from build123d import *

# Parameters (mm, degrees)
SKETCH_1_W           = 2.4
SKETCH_1_H           = 2.4
EXTRUDE_1_DEPTH      = 7.2
EXTRUDE_2_DEPTH      = 18
EXTRUDE_2_DEPTH_BACK = 12
SKETCH_4_W           = 2.3
SKETCH_4_H           = 2.3
EXTRUDE_3_DEPTH      = 7
EXTRUDE_3_DEPTH_BACK = 2.3
SKETCH_5_R           = 0.35
SKETCH_6_R           = 0.35
CUT_EXTRUDE_1_DEPTH  = 10
FILLET_1_SIZE        = 2.4
FILLET_1_SIZE_2      = 3.2
FILLET_2_R           = 0.5
EXTRUDE_START        = -1.5
SKETCH_7_W           = 1.15
SKETCH_7_H           = 0.45
SKETCH_7_H_2         = 1.3
SKETCH_7_H_3         = 2.2
EXTRUDE_4_DEPTH      = 5.1
SKETCH_8_W           = 7.2
SKETCH_8_H           = 2.2
EXTRUDE_5_DEPTH      = 3.1


with BuildPart() as part:
    # 草图1 → 凸台-拉伸1 (new body)
    with BuildSketch(Plane.XY):
        Rectangle(SKETCH_1_W, SKETCH_1_H)
    extrude(amount=EXTRUDE_1_DEPTH)

    # 草图4 → 凸台-拉伸2 (add, two sides: drawn at the far end of the back side and taken through both)
    with BuildSketch(Plane(origin=(0, 0, 0), x_dir=(0, 0, -1), z_dir=(1, 0, 0)).offset(-EXTRUDE_2_DEPTH_BACK)):
        Rectangle(SKETCH_4_W, SKETCH_4_H)
    extrude(amount=EXTRUDE_2_DEPTH + EXTRUDE_2_DEPTH_BACK)

    # 草图5 → 凸台-拉伸3 (add, two sides: drawn at the far end of the back side and taken through both)
    with BuildSketch(Plane.XY.offset(1.15).offset(-EXTRUDE_3_DEPTH_BACK)):
        with BuildLine():
            Line((18, 0), (18, 1.15))
            Line((18, 1.15), (19.15, 1.15))
            ThreePointArc((19.15, 1.15), (20.3, 0), (19.15, -1.15))
            Line((19.15, -1.15), (18, -1.15))
            Line((18, -1.15), (18, 0))
        make_face()
        with Locations(Location((19.15, 0, 0), (0, 0, 180))):
            Circle(SKETCH_5_R, mode=Mode.SUBTRACT)
    extrude(amount=EXTRUDE_3_DEPTH + EXTRUDE_3_DEPTH_BACK)

    # 草图6 → 切除-拉伸1 (cut)
    with BuildSketch(Plane.ZY.offset(12)):
        Circle(SKETCH_6_R)
    extrude(amount=-CUT_EXTRUDE_1_DEPTH, mode=Mode.SUBTRACT)

    # 圆角1
    # an asymmetric fillet: 3.2, 2.4 mm, written as the material it adds along each edge
    with BuildSketch(Plane(origin=(18, 1.15, 1.15), x_dir=(-1, 0, 0), z_dir=(0, -1, 0))) as fillet_1_piece_1:
        with BuildLine():
            Bezier((FILLET_1_SIZE, 0), (0, 0), (0, -FILLET_1_SIZE_2), weights=[1, 0.707106781, 1])
            Line((0, -FILLET_1_SIZE_2), (0, 0))
            Line((0, 0), (FILLET_1_SIZE, 0))
        make_face()
    extrude(amount=2.3)

    # 圆角2
    fillet_2_edges = [part.edges().sort_by_distance(p)[0] for p in [
        (-6.6, -1.15, 1.15),
        (3.575, -1.15, -1.15),
        (-6.6, 1.15, 1.15),
        (3.575, 1.15, -1.15),
        (20.3, 0, -1.15),
    ]]
    fillet(fillet_2_edges, radius=FILLET_2_R)

    # 草图7 → 凸台-拉伸4 (add)
    with BuildSketch(Plane.XY.offset(1.15).offset(EXTRUDE_START)):
        with Locations((-3.025, 0.875)):
            Rectangle(SKETCH_7_W, SKETCH_7_H)
        with Locations((-3.025, 0)):
            Rectangle(SKETCH_7_W, SKETCH_7_H_2)
        with Locations((-3.025, -0.875)):
            Rectangle(SKETCH_7_W, SKETCH_7_H)
        with Locations((3.025, 0)):
            Rectangle(SKETCH_7_W, SKETCH_7_H_3)
    extrude(amount=EXTRUDE_4_DEPTH)

    # 草图8 → 凸台-拉伸5 (add)
    with BuildSketch(Plane.XY.offset(1.15).offset(EXTRUDE_START)):
        Rectangle(SKETCH_8_W, SKETCH_8_H)
    extrude(amount=EXTRUDE_5_DEPTH)


solid = part.part
Can you work these out from the model? Positions are in its coordinate system, mm. A direction names the side the tool comes from. Give positions to 0.01 mm unless a question says otherwise; leave off trailing zeros. Order: outer loops, then holes, each group sorted by start corner. A loop starts at its lowest first (then second) coordinate and runs counter-clockwise, first axis right, second up. Notation, with made-up numbers: M 9.5,61 L 37.5,61 A26 ccw 37.5,94 Z; hole C 26,-3 d1. An arc over 180 degrees is marked long. One line per item, written item: value.
Item 1: If we section it at A-A on z = 6.75: Write out the boundary of the cut face in (x, y), and give its area (3 significant figures).
Verdict:
outline: M -1.2,-1.2 L 1.2,-1.2 L 1.2,1.2 L -1.2,1.2 Z; M 18,-1.15 L 19.15,-1.15 A1.15 ccw 19.15,1.15 L 18,1.15 Z; hole C 19.15,0 d0.7
area: 10.1 mm2
Item 2: Please list where these lines run through material, in increasing order: line 1 (Y direction, x = 19.15, z = 5); line 2 (X direction, y = 0.45, z = 4.5).
Verdict:
line 1: -1.15 to -0.35, 0.35 to 1.15
line 2: -3.6 to -2.45, -1.2 to 1.2, 2.45 to 3.6, 18 to 20.21
Item 3: If we section it at B-B on x = -0.5: Write out the boundary of the cut face in (y, z).
Verdict:
outline: M -1.2,0 L -1.15,0 L -1.15,-0.65 A0.5 ccw -0.65,-1.15 L 0.65,-1.15 A0.5 ccw 1.15,-0.65 L 1.15,0 L 1.2,0 L 1.2,7.2 L -1.2,7.2 Z
Item 4: If we section it at D-D on z = 3.25: State how many separate pieces and enclosed holes the cut face has, and give its area (3 significant figures).
Verdict:
separate pieces: 4
enclosed holes: 1
area: 15.5 mm2
Item 5: For pin 1 (0.7 mm diameter, centred on x = 2.5, z = 3, fed in from -Y); pin 2 (0.7 mm diameter, centred on y = -0.5, z = 6.5, fed in from -X); pin 3 (0.8 mm diameter, centred on y = 0, z = 0, fed in from -X); pin 4 (1 mm diameter, centred on x = -4, z = 2.5, fed in from +Y), each with a flat end and sliding along its axis, tell me the tip position at first contact or that it passes through.
Verdict:
pin 1: y = -1.1
pin 2: x = -1.2
pin 3: x = -12
pin 4: y = 1.1
Item 6: If we mould it in two halves opening along X, with no side actions, what happens to faces 6 (the face through (-8, 0, 1.15)), 7 (the face through (-3.6, 0, 3)), 8 (the face through (18, 0, 6)), 9 (the face through (20.3, 0, 3.7))? For each: pulls with the +X half, pulls with the -X half, needs draft (parallel to the pull), parting line crosses it, or undercut.
Verdict:
face 6: needs draft
face 7: pulls with the -X half
face 8: undercut
face 9: pulls with the +X half
Item 7: If we section it at C-C on x = -8.5: Write out the boundary of the cut face in (y, z).
Verdict:
outline: M -1.15,-0.65 A0.5 ccw -0.65,-1.15 L 0.65,-1.15 A0.5 ccw 1.15,-0.65 L 1.15,0.65 A0.5 ccw 0.65,1.15 L -0.65,1.15 A0.5 ccw -1.15,0.65 Z; hole C 0,0 d0.7
Item 8: For faces 1 (the face through (-3, -1.1, 2)), 2 (the face through (3, 1.1, 3)), 3 (the face through (-2, 0, 2.75)), 4 (the face through (0, 0, 7.2)), 5 (the face through (-3, 1.1, 2)), which set-ups out of +Z, -Z, +X, -X, +Y, -Y let a thin tool reach every point of the face, with its end or its side?
Verdict:
face 1: +Z, -X, -Y
face 2: +Z, +Y
face 3: +Z, +Y, -Y
face 4: +Z, -X, +Y, -Y
face 5: +Z, -X, +Y
